```python
from build123d import *

# Parameters (mm, degrees)
SKETCH_1_W      = 50
SKETCH_1_H      = 1
EXTRUDE_1_DEPTH = 10
SKETCH_2_W      = 10
SKETCH_2_H      = 1.5
EXTRUDE_2_DEPTH = 15
FILLET_3_R      = 0.5


with BuildPart() as part:
    # 草图1 → 凸台-拉伸1 (new body)
    with BuildSketch(Plane.XY):
        with Locations((25, 0.5)):
            Rectangle(SKETCH_1_W, SKETCH_1_H)
    extrude(amount=EXTRUDE_1_DEPTH)

    # 草图2 → 凸台-拉伸2 (add)
    with BuildSketch(Plane(origin=(0, 1, 0), x_dir=(1, 0, 0), z_dir=(0, 1, 0))):
        with Locations((13, -2.45)):
            Rectangle(SKETCH_2_W, SKETCH_2_H)
        with Locations((24.5, -2.45)):
            Rectangle(SKETCH_2_W, SKETCH_2_H)
        with Locations((36, -2.45)):
            Rectangle(SKETCH_2_W, SKETCH_2_H)
    extrude(amount=EXTRUDE_2_DEPTH)

    # 圆角3
    fillet_3_edges = [part.edges().sort_by_distance(p)[0] for p in [
        (25, 1, 10),
        (8, 1, 2.45),
        (8, 8.5, 1.7),
        (13, 1, 3.2),
        (8, 8.5, 3.2),
        (18, 1, 2.45),
        (18, 8.5, 3.2),
        (13, 1, 1.7),
        (18, 8.5, 1.7),
        (8, 16, 2.45),
        (13, 16, 3.2),
        (18, 16, 2.45),
        (13, 16, 1.7),
        (19.5, 1, 2.45),
        (19.5, 8.5, 1.7),
        (24.5, 1, 3.2),
        (19.5, 8.5, 3.2),
        (29.5, 1, 2.45),
        (29.5, 8.5, 3.2),
        (24.5, 1, 1.7),
        (29.5, 8.5, 1.7),
        (19.5, 16, 2.45),
        (24.5, 16, 3.2),
        (29.5, 16, 2.45),
        (24.5, 16, 1.7),
        (31, 1, 2.45),
        (31, 8.5, 1.7),
        (36, 1, 3.2),
        (31, 8.5, 3.2),
        (41, 1, 2.45),
        (41, 8.5, 3.2),
        (36, 1, 1.7),
        (41, 8.5, 1.7),
        (31, 16, 2.45),
        (36, 16, 3.2),
        (41, 16, 2.45),
        (36, 16, 1.7),
        (25, 1, 0),
        (0, 1, 5),
        (50, 1, 5),
    ]]
    fillet(fillet_3_edges, radius=FILLET_3_R)


solid = part.part
```
Input: part model. Units: mm. Frame: model coordinates. A direction names the side the tool comes from. Round coordinates to 2 decimals unless told otherwise and drop trailing zeros. Loops run counter-clockwise (first coordinate to the right, second up) from the corner with the lowest first, then second, coordinate; pieces in that order, holes last. Notation, with made-up numbers: (48.5, 28) -> (107.5, 28) arc R18 ccw to (107.5, 39) -> close; hole circle Ø9 at (30, 24.5). An arc over 180 degrees is marked (long way). Use one line per item in the form item = value. Start each with the question number.
Item 1: Mould query, pull axis Z, two halves, no side actions, for faces 1 (the face through (24, 8, 1.7)), 2 (the face through (36, 8, 3.2)), 3 (the face through (25, 0, 5)). Classes: pulls with the +Z half, pulls with the -Z half, needs draft (parallel to the pull), parting line crosses it, or undercut.
Item 2: Section query B-B on x = 14. Return the cut outline in (y, z), then the cut area to 3 significant figures.
Item 3: Contact query for flat-ended pins moving along their axis: pin 1 Ø5 at (x, y) = (11.5, 9) entering from -Z; pin 2 Ø2.5 at (x, y) = (36, 10.5) entering from +Z; pin 3 Ø2 at (y, z) = (6.5, 2) entering from +X. Output: stop coordinate, or through.
Item 4: Set-up query: faces 4 (the face through (13, 8, 1.7)), 5 (the face through (13, 8, 3.2)). Return all of +Z, -Z, +X, -X, +Y, -Y with unobstructed straight access to the full face (end or side cutting, diameter ignored); none if empty.
Item 5: Material intervals for L1, parallel to X at y = 9.25, z = 2.75; L2, parallel to X at y = 7, z = 3; L3, parallel to Y at x = 43, z = 8.75, sorted ascending. Write a range as from..to.
Item 6: Section query A-A on y = 7.75. Return the cut outline in (x, z).
Item 7: Section query C-C on z = 7.5. Return the cut outline in (x, y).
Ans:
q1.face_1 = pulls with the -Z half
q1.face_2 = pulls with the +Z half
q1.face_3 = needs draft
q2.outline = (0, 0) -> (0.5, 0) arc R0.5 ccw to (1, 0.5) -> (1, 1.2) arc R0.5 cw to (1.5, 1.7) -> (15.5, 1.7) arc R0.5 ccw to (16, 2.2) -> (16, 2.7) arc R0.5 ccw to (15.5, 3.2) -> (1.5, 3.2) arc R0.5 cw to (1, 3.7) -> (1, 9.5) arc R0.5 ccw to (0.5, 10) -> (0, 10) -> close
q2.area = 32.4 mm^2
q3.pin_1 = 1.7
q3.pin_2 = 3.2
q3.pin_3 = 41
q4.face_4 = -Z, +X, -X, +Y
q4.face_5 = +Z, +X, -X, +Y
q5.L1 = 8..18, 19.5..29.5, 31..41
q5.L2 = 8.1..17.9, 19.6..29.4, 31.1..40.9
q5.L3 = 0..1
q6.outline = (8, 2.2) arc R0.5 ccw to (8.5, 1.7) -> (17.5, 1.7) arc R0.5 ccw to (18, 2.2) -> (18, 2.7) arc R0.5 ccw to (17.5, 3.2) -> (8.5, 3.2) arc R0.5 ccw to (8, 2.7) -> close; (19.5, 2.2) arc R0.5 ccw to (20, 1.7) -> (29, 1.7) arc R0.5 ccw to (29.5, 2.2) -> (29.5, 2.7) arc R0.5 ccw to (29, 3.2) -> (20, 3.2) arc R0.5 ccw to (19.5, 2.7) -> close; (31, 2.2) arc R0.5 ccw to (31.5, 1.7) -> (40.5, 1.7) arc R0.5 ccw to (41, 2.2) -> (41, 2.7) arc R0.5 ccw to (40.5, 3.2) -> (31.5, 3.2) arc R0.5 ccw to (31, 2.7) -> close
q7.outline = (0, 0) -> (50, 0) -> (50, 0.5) arc R0.5 ccw to (49.5, 1) -> (0.5, 1) arc R0.5 ccw to (0, 0.5) -> close
